Geometry check sheet. Reference: drawing and pictorial views, mm from the part's lowest x, y, z. A direction names the side the tool comes from. Give positions to 0.01 mm unless a question says otherwise; leave off trailing zeros. Order: outer loops, then holes, each group sorted by start corner. A loop starts at its lowest first (then second) coordinate and runs counter-clockwise, first axis right, second up.
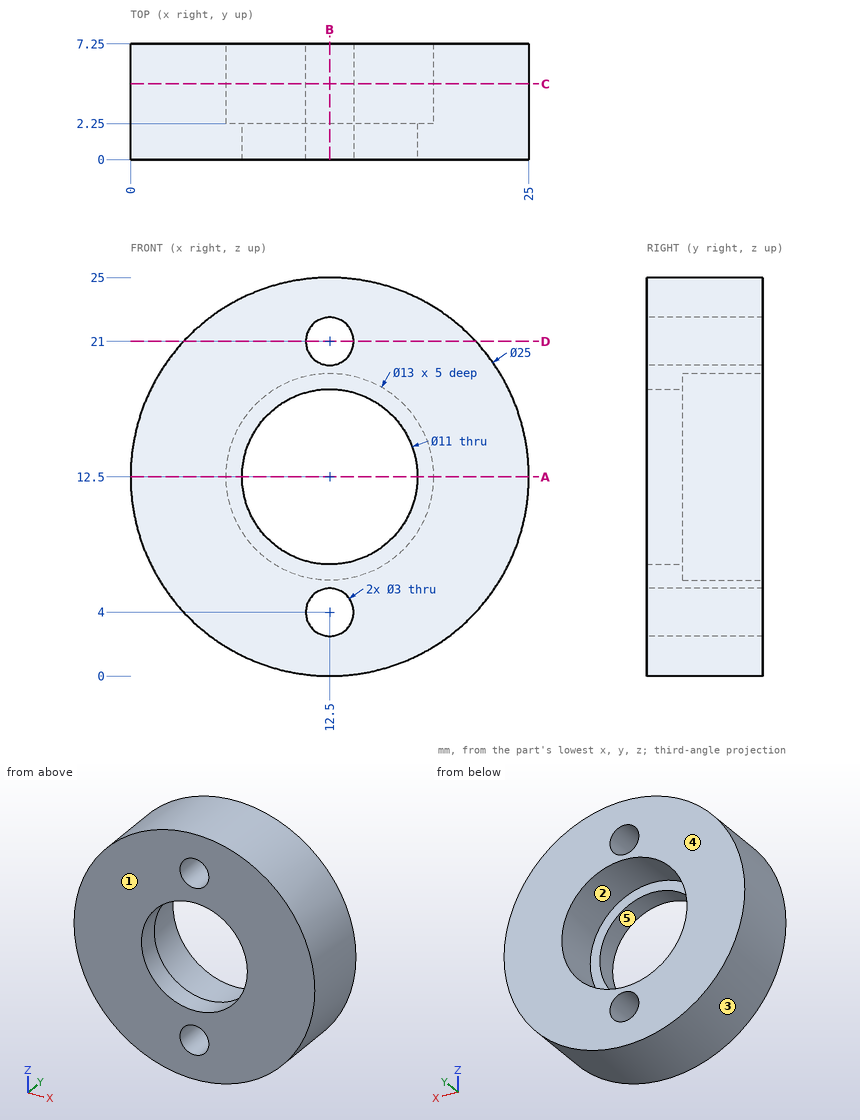
(1) Cross-section at B-B on x = 12.5. Enter the section's corners in (y, z), then the cut area to 3 significant figures.
Response values:
outline: (0, 0) - (7.25, 0) - (7.25, 2.5) - (0, 2.5) - close; (0, 5.5) - (7.25, 5.5) - (7.25, 6) - (2.25, 6) - (2.25, 7) - (0, 7) - close; (0, 18) - (2.25, 18) - (2.25, 19) - (7.25, 19) - (7.25, 19.5) - (0, 19.5) - close; (0, 22.5) - (7.25, 22.5) - (7.25, 25) - (0, 25) - close
area: 48.0 mm2
(2) Material ranges on L1, parallel to Z at x = 12.5, y = 1.05; L2, parallel to Z at x = 12.5, y = 4.5; L3, parallel to X at y = 1.5, z = 12.5, recorded low to high.
Response values:
L1: z = 0 to 2.5, 5.5 to 7, 18 to 19.5, 22.5 to 25
L2: z = 0 to 2.5, 5.5 to 6, 19 to 19.5, 22.5 to 25
L3: x = 0 to 7, 18 to 25
(3) Release check for a two-part mould opening along Z. For the marked faces 3, 4 and 5 record: released by +Z, released by -Z, zero draft, split by the parting line, or undercut.
Response values:
face 3: split by the parting line
face 4: zero draft
face 5: undercut
(4) Cross-section at C-C on y = 4.75. Enter the section's corners in (x, z), then the cut area to 3 significant figures.
Response values:
outline: circle Ø25 at (12.5, 12.5); hole circle Ø13 at (12.5, 12.5); hole circle Ø3 at (12.5, 4); hole circle Ø3 at (12.5, 21)
area: 344 mm2
(5) Set-up check for the marked faces 1 and 2: record each of +Z, -Z, +X, -X, +Y, -Y from which the full face is reachable in a straight line by a thin tool's end or side.
Response values:
face 1: +Z, -Z, +X, -X, -Y
face 2: +Y
(6) Cross-section at A-A on z = 12.5. Enter the section's corners in (x, y).
Response values:
outline: (0, 0) - (7, 0) - (7, 2.25) - (6, 2.25) - (6, 7.25) - (0, 7.25) - close; (18, 0) - (25, 0) - (25, 7.25) - (19, 7.25) - (19, 2.25) - (18, 2.25) - close
(7) Cross-section at D-D on z = 21. Enter the section's corners in (x, y), then the cut area to 3 significant figures.
Response values:
outline: (3.33, 0) - (11, 0) - (11, 7.25) - (3.33, 7.25) - close; (14, 0) - (21.67, 0) - (21.67, 7.25) - (14, 7.25) - close
area: 111 mm2
(8) Gauge pin test, flat ends, axial feed: pin 1 Ø2 at (y, z) = (4, 19) entering from -X (3 decimals); pin 2 Ø3 at (x, y) = (16, 1.5) entering from -Z; pin 3 Ø4 at (x, z) = (14.5, 9.5) entering from +Y. Record the tip position at first contact, or that the pin passes through.
Response values:
pin 1: stops at x = 1.275
pin 2: stops at z = 0.16
pin 3: stops at y = 2.25
